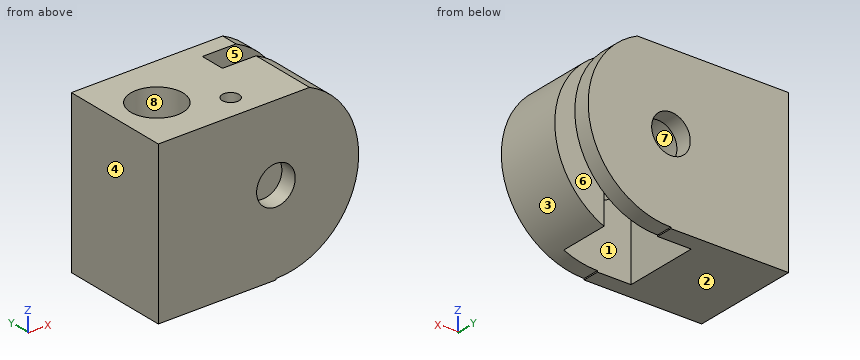
Autodesk Inventor part; units mm, degrees
ref_plane "YZ Plane" through (0, 0, 0) normal (1, 0, 0) x (0, 1, 0)
ref_plane "XZ Plane" through (0, 0, 0) normal (0, 1, 0) x (-1, 0, 0)
ref_plane "XY Plane" through (0, 0, 0) normal (0, 0, 1) x (1, 0, 0)
sketch "スケッチ1" plane through (0, 0, 0) normal (0, 1, 0) x (-1, 0, 0)
  circle A0 centre (0, 0) radius 1.15
  circle A1 centre (0, 0) radius 2
  circle A2 centre (0, 0) radius 5
  line L0 (0, 0) -> (7, 0)
  line L1 (7, 0) -> (7, 4.5)
  line L2 (7, 4.5) -> (0, 4.5)
  line L3 (0, 4.5) -> (0, 0)
  line L4 (0, 0) -> (7, 0)
  line L5 (7, 0) -> (7, -5)
  line L6 (7, -5) -> (0, -5)
  line L7 (0, -5) -> (0, 0)
  line L8 (0, 4.5) -> (-2, 4.5)
  line L9 (-2, 4.5) -> (-2, 0)
  line L10 (-2, 0) -> (0, 0)
  line L11 (0, 0) -> (0, 4.5)
  circle A3 centre (0, 0) radius 3
  line L12 (-2, 0) -> (-2, -5)
  line L13 (-2, -5) -> (0, -5)
  line L14 (2, 0) -> (2, -5)
  circle A4 centre (0, 0) radius 4.9244
  line L15 (-2, 0) -> (-4.9244, 0)
  point P0 (0, 2)
  point P1 (-2, 2.2361)
  point P2 (-2, -2.2361)
  point P3 (-2, -4.5826)
  point P4 (-2, -4.5)
  point P5 (0, -4.9244)
  dimension "d2" = 10
  dimension "d0" = 2.3
  dimension "d1" = 4
  dimension "d3" = 7
  dimension "d4" = 4.5
  dimension "d5" = 6
extrude "押し出し1" add sketch "スケッチ1" along normal blind 4.5 contours A1 L3 A3 L0 | L0 A3 L14 | A3 L3 L2 A4 L0 | L0 A4 L14 A3 | A4 L2 A2 L0 | L0 A2 L14 A4 | L0 L5 L6 L14 A2 | A2 L2 L1 L0
extrude "押し出し2" add sketch "スケッチ1" along normal blind 3 contours A1 L9 A3 L3 | L15 A3 L9 | L12 A3 L15 | A3 L9 L8 L3 | A3 L15 A4 L9 | L12 A4 L15 A3
extrude "押し出し3" add sketch "スケッチ1" against normal blind 1 contours L0 A1 L7 A0 | A0 L3 A1 L0 | A0 L10 A1 L3 | L7 A1 L10 A0 | L14 A3 L7 A1 | A1 L3 A3 L0 | L0 A3 L14 | A1 L9 A3 L3 | L7 A3 L12 A1 | A3 L3 L2 A4 L0 | L0 A4 L14 A3 | L14 A4 L7 A3 | L15 A3 L9 | L12 A3 L15 | A3 L9 L8 L3 | L7 A4 L12 A3 | A4 L2 A2 L0 | L0 A2 L14 A4 | L14 A2 L7 A4 | A3 L15 A4 L9 | L12 A4 L15 A3 | L0 L5 L6 L14 A2 | A2 L2 L1 L0 | L14 L6 A2
sketch "スケッチ2" plane through (0, 4.5, 0) normal (0, 1, 0) x (1, 0, 0)
  circle A0 centre (0, 0) radius 1.15
  circle A1 centre (0, 0) radius 2
  circle A2 centre (0, 0) radius 4.9244
  line L0 (0, 0) -> (2, 0)
  line L1 (2, 0) -> (2, -4.5)
  line L2 (2, -4.5) -> (0, -4.5)
  line L3 (0, -4.5) -> (0, 0)
  line L4 (-2, 5) -> (-7, 5)
  line L5 (0, -4.5) -> (-7, -4.5)
  line L6 (-7, -4.5) -> (-7, 5)
  line L7 (-7, 5) -> (0, 5)
  line L8 (0, 5) -> (0, -4.5)
  line L9 (0, 0) -> (2, 0)
  line L10 (2, 0) -> (2, 5)
  line L11 (2, 5) -> (0, 5)
  line L12 (0, 5) -> (0, 0)
  point P0 (0, 4.9244)
  dimension "d12" = 4
extrude "押し出し4" add sketch "スケッチ2" along normal blind 1 contours L0 A1 L3 A0 | A0 L8 A1 L0 | A0 L3 A1 L8 | L1 L2 L3 A1 | L10 A2 L1 | A1 L8 A2 L10 | A1 L3 L5 A2 L8 | A2 L5 L6 L4 L7 L8
sketch "スケッチ3" plane through (0, 3, 4.5) normal (0, 0, 1) x (1, 0, 0)
  line L0 (-7, -4) -> (-7, 2.5)
  line L1 (-7, 2.5) -> (-4.5, 2.5)
  line L2 (-4.5, 2.5) -> (-4.5, -0.75)
  line L3 (-4.5, -0.75) -> (-7, -0.75)
  line L4 (-7, -0.75) -> (-7, 2.5)
  circle A0 centre (-4.5, -0.75) radius 1.55
  line L5 (0, -3) -> (-2, -3)
  line L6 (0, -3) -> (-1.5, -3)
  line L7 (-1.5, -3) -> (-1.5, -2.5)
  line L8 (-1.5, -2.5) -> (0, -2.5)
  line L9 (0, -2.5) -> (0, -3)
  circle A1 centre (-1.5, -2.5) radius 0.5
  dimension "d15" = 2.5
  dimension "d16" = 3.25
  dimension "d17" = 3.1
  dimension "d18" = 1.5
  dimension "d19" = 0.5
extrude "押し出し5" cut sketch "スケッチ3" against normal blind 8 contours A0 L2 L3 | L3 L2 A0 | A1 L8 L7 | L7 L8 A1
properties part number "rod5.1"
Source: CAD feature listing. Evaluate the final solid. Frame: model axes, mm. Face numbers are marked on the shaded views. A direction names the side the tool comes from. Round coordinates to 2 decimals unless told otherwise and drop trailing zeros. Loops run counter-clockwise (first coordinate to the right, second up) from the corner with the lowest first, then second, coordinate; pieces in that order, holes last. Notation, with made-up numbers: (16, -30.75) - (29, -30.75) arc R26 ccw to (29, -16.75) - close; hole circle Ø8 at (37.25, 16.5). An arc over 180 degrees is marked (long way). Write item = value, one per line. Start each with the question number.
(1) Pin query (flat end, axial travel): pin 1 (2 mm diameter, centred on y = 3.5, z = -2, fed in from +X); pin 2 (0.8 mm diameter, centred on y = 4, z = 3.5, fed in from +X); pin 3 (2.5 mm diameter, centred on x = -4, y = 2.5, fed in from +Z); pin 4 (1.8 mm diameter, centred on x = 0, z = 0, fed in from +Y). Return the tip coordinate at first contact, or that it passes through.
(2) Set-up query: the marked faces 5, 6, 7 and 8. Return all of +Z, -Z, +X, -X, +Y, -Y with unobstructed straight access to the full face (end or side cutting, diameter ignored); none if empty.
(3) Section query B-B, the plane x = -4.5. Output: boundary loops of the cut face in (y, z).
(4) Section query A-A, the plane z = -0.75. Output: boundary loops of the cut face in (x, y), plus the area to 3 significant figures.
(5) Section query C-C, the plane z = 4. Output: boundary loops of the cut face in (x, y), plus the area to 3 significant figures.
(6) Pull-direction query (X, two-part tool) for the marked faces 1, 2, 3 and 4; classes: +X half, -X half, draft (parallel to the pull), parting line (faces both ways), or undercut.
(7) Section query D-D, the plane y = 3.5. Output: boundary loops of the cut face in (x, z).
(8) Ray query, line 1 along Y through (x, z) = (-4.5, 3); line 2 along Y through (x, z) = (1.75, 3); line 3 along X through (y, z) = (4.7, 0). Return the intervals inside material, ascending. Write a range as from..to.
Conclusion:
q1.pin_1 = 4.79
q1.pin_2 = 0
q1.pin_3 = 4.5
q1.pin_4 = through
q2.face_5 = -Z, +X
q2.face_6 = +Z, -Z, +X
q2.face_7 = -Z
q2.face_8 = +Z
q3.outline = (-1, -5) - (5.5, -5) - (5.5, 4.5) - (3.8, 4.5) - (3.8, -3.5) - (0.7, -3.5) - (0.7, 4.5) - (-1, 4.5) - close
q4.outline = (-7, -1) - (-0.87, -1) - (-0.87, 0) - (-2, 0) - (-2, 4.5) - (-0.87, 4.5) - (-0.87, 5.5) - (-7, 5.5) - close; (0.87, -1) - (4.87, -1) - (4.87, 3) - (2, 3) - (2, 0) - (0.87, 0) - close; (0.87, 4.5) - (4.87, 4.5) - (4.87, 5.5) - (0.87, 5.5) - close; hole circle Ø3.1 at (-4.5, 2.25)
q4.area = 43.8 mm2
q5.outline = (-7, -1) - (2.87, -1) - (2.87, 3) - (0, 3) - (0, 4.5) - (2.87, 4.5) - (2.87, 5.5) - (-7, 5.5) - close; hole circle Ø3.1 at (-4.5, 2.25); hole circle Ø1 at (-1.5, 0.5)
q5.area = 51.5 mm2
q6.face_1 = undercut
q6.face_2 = draft
q6.face_3 = +X half
q6.face_4 = -X half
q7.outline = (-7, -5) - (-2, -5) - (-2, 0) arc R2 cw to (0, 2) - (0, 4.5) - (-3.58, 4.5) - (-3.58, -3.5) - (-5.42, -3.5) - (-5.42, 4.5) - (-7, 4.5) - close
q8.line_1 = -1..0.7, 3.8..5.5
q8.line_2 = -1..3, 4.5..5.5
q8.line_3 = -7..-1.15, 1.15..4.92
